Autodesk Inventor part; units mm, degrees
ref_plane "YZ Plane" through (0, 0, 0) normal (1, 0, 0) x (0, 1, 0)
ref_plane "XZ Plane" through (0, 0, 0) normal (0, 1, 0) x (-1, 0, 0)
ref_plane "XY Plane" through (0, 0, 0) normal (0, 0, 1) x (1, 0, 0)
sketch "Sketch1" plane through (0, 0, 0) normal (0, 1, 0) x (-1, 0, 0)
  arc A0 (176.3419, -210.5927) -> (175.3044, -30.5987) centre (175.3044, -120.5987) ccw
  line L0 (175.3044, -30.5987) -> (91.4725, -30.5987)
  line L1 (-2.1956, -66.2894) -> (-2.1956, -174.8751)
  line L2 (91.4505, -210.5927) -> (176.3419, -210.5927)
  arc A1 (44.9453, -8.483) -> (-6.6956, -55.5772) centre (17.8044, -30.5822) ccw
  arc A2 (-6.6956, -185.5872) -> (44.9372, -232.6914) centre (17.8044, -210.5822) ccw
  line L3 (265.3044, -138.5987) -> (263.4861, -138.5987)
  line L4 (263.4861, -102.5987) -> (265.3044, -102.5987)
  circle A3 centre (175.3044, -120.5987) radius 14.5
  line L5 (175.3044, -52.5987) -> (77.8044, -52.5987)
  line L6 (77.8044, -188.5987) -> (175.3044, -188.5987)
  arc A4 (237.9792, -94.2194) -> (175.3044, -52.5987) centre (175.3044, -120.5987) ccw
  arc A5 (175.3044, -188.5987) -> (237.9792, -146.978) centre (175.3044, -120.5987) ccw
  line L7 (228.7624, -133.0987) -> (217.1374, -133.0987)
  line L8 (217.1374, -108.0987) -> (228.7624, -108.0987)
  line L9 (139.9491, -108.0987) -> (106.0335, -108.0987)
  line L10 (106.0335, -133.0987) -> (139.9491, -133.0987)
  arc A6 (208.3305, -102.8356) -> (139.9491, -108.0987) centre (175.3044, -120.5987) ccw
  arc A7 (139.9491, -133.0987) -> (208.3305, -138.3619) centre (175.3044, -120.5987) ccw
  line L11 (62.8044, -67.5987) -> (62.8044, -62.504)
  line L12 (62.8044, -178.6935) -> (62.8044, -173.5987)
  arc A8 (106.0335, -108.0987) -> (74.0544, -77.0277) centre (62.8044, -120.5987) ccw
  arc A9 (74.0544, -164.1698) -> (106.0335, -133.0987) centre (62.8044, -120.5987) ccw
  circle A10 centre (62.8044, -120.5987) radius 21
  circle A11 centre (17.8044, -30.5822) radius 21
  circle A12 centre (17.8044, -210.5822) radius 21
  arc A13 (239.6919, -108.0987) -> (241.6431, -105.6593) centre (239.6919, -106.0987) ccw
  arc A14 (228.7624, -108.0987) -> (237.9792, -94.2194) centre (228.7624, -98.0987) ccw
  arc A15 (208.3305, -102.8356) -> (217.1374, -108.0987) centre (217.1374, -98.0987) ccw
  arc A16 (217.1374, -133.0987) -> (208.3305, -138.3619) centre (217.1374, -143.0987) ccw
  arc A17 (237.9792, -146.978) -> (228.7624, -133.0987) centre (228.7624, -143.0987) ccw
  arc A18 (77.8044, -52.5987) -> (62.8044, -67.5987) centre (77.8044, -67.5987) ccw
  arc A19 (62.8044, -173.5987) -> (77.8044, -188.5987) centre (77.8044, -173.5987) ccw
  arc A20 (62.8044, -62.504) -> (74.0544, -77.0277) centre (77.8044, -62.504) ccw
  arc A21 (74.0544, -164.1698) -> (62.8044, -178.6935) centre (77.8044, -178.6935) ccw
  arc A22 (44.9453, -8.483) -> (91.4725, -30.5987) centre (91.4725, 29.4013) ccw
  arc A23 (91.4505, -210.5927) -> (44.9372, -232.6914) centre (91.4505, -270.5927) ccw
  arc A24 (-2.1956, -66.2894) -> (-6.6956, -55.5772) centre (-17.1956, -66.2894) ccw
  arc A25 (-6.6956, -185.5872) -> (-2.1956, -174.8751) centre (-17.1956, -174.8751) ccw
  point P0 (0, 0)
  point P1 (-2.1956, -181.8594)
  point P2 (242.1457, -108.0987)
  point P3 (242.1457, -133.0987)
  point P4 (62.8044, -188.5987)
  point P5 (210.6598, -108.0987)
  point P6 (210.6598, -133.0987)
  point P7 (62.8044, -52.5987)
  point P8 (62.8044, -75.5987)
  point P9 (62.8044, -165.5987)
  point P10 (-2.1956, -59.3051)
  point P11 (52.8044, -30.5987)
  point P12 (52.8044, -210.5927)
  point P13 (63.0223, -65.0513)
  point P14 (63.0223, -176.1461)
  dimension "d0" = 180
  dimension "d1" = 20
  dimension "d2" = 20
  dimension "d3" = 42
  dimension "d4" = 70
  dimension "d5" = 42
  dimension "d6" = 70
  dimension "d7" = 112.5
  dimension "d8" = 90
  dimension "d9" = 90
  dimension "d10" = 25
  dimension "d11" = 90
  dimension "d12" = 68
  dimension "d13" = 77.5
  dimension "d14" = 37.5
  dimension "d15" = 37.5
  dimension "d16" = 29
  dimension "d17" = 45
  dimension "d18" = 45
  dimension "d19" = 42
  dimension "d20" = 25
  dimension "d21" = 77.5
  dimension "d22" = 112.5
  dimension "d23" = 112.5
  dimension "d24" = 45
  dimension "d25" = 68
  dimension "d26" = 2
  dimension "d27" = 10
  dimension "d28" = 15
  dimension "d29" = 60
extrude "Extrusion1" add sketch "Sketch1" along normal blind 10
equation "\"d2\" = d1"
equation "\"d5\" = d3"
equation "\"d6\" = d4"
equation "\"d15\" = d14"
equation "\"d18\" = d17"
equation "\"d20\" = d10"
equation "\"d21\" = d13"
equation "\"d25\" = d12"
For this review, take the finished solid that the model builds, in its own axes (mm). A direction names the side the tool comes from. Give positions to 0.01 mm unless a question says otherwise; leave off trailing zeros. Order: outer loops, then holes, each group sorted by start corner. A loop starts at its lowest first (then second) coordinate and runs counter-clockwise, first axis right, second up. Notation, with made-up numbers: (-13.75, 64.25) - (24.25, 64.25) arc R22 ccw to (24.25, 70.25) - close; hole circle Ø7 at (-19.5, 62). An arc over 180 degrees is marked (long way). Answer as a JSON object with one key per item and string values. Group by question number.
Item 1: Clearance check with flat-ended pins moving along their axes: pin 1 Ø5 at (x, y) = (-122, 7) entering from -Z; pin 2 Ø6 at (y, z) = (4, -91.5) entering from +X; pin 3 Ø1 at (x, y) = (-59.5, 3) entering from -Z. State where each tip first meets the part, or that it passes through.
Item 2: Machinability: for faces 1 (the flat face through (-223, 5, -133.099)), 2 (the cylindrical face through (-65.366, 4.93, -216.559)), 3 (the cylindrical face through (3.334, 4.93, -180.607)), 4 (the flat face through (-134, 5, -30.599)), which of the approach directions +Z, -Z, +X, -X, +Y, -Y give a long, thin tool a straight path to every point of the face, cutting with its end or side? Answer none if there is none.
Item 3: Wall thickness on line 1 along Z through (x, y) = (-112, 8.75); line 2 along X through (y, z) = (6, -106); line 3 along Z through (x, y) = (-232.5, 1.75): over which ranges is each line inside the solid? List them lowest first.
Item 4: Take a section at A-A on x = -150. Give the boundary of the cut face in (y, z), and give its area (3 significant figures).
Item 5: Draft analysis for pull direction Z (two halves, no side actions). For faces 5 (the flat face through (-91, 10, -119)), 6 (the cylindrical face through (3.4, 4.9, -60.4)), 7 (the cylindrical face through (-265.27, 4.93, -118.11)), state which applies: pulls with the +Z half, pulls with the -Z half, needs draft (parallel to the pull), parting line crosses it, or undercut.
Item 6: Take a section at B-B on z = -151. Give the boundary of the cut face in (x, y).
Item 7: Take a section at C-C on z = -25. Give the boundary of the cut face in (x, y), and give its area (3 significant figures).
Reported:
{
 "1": {"pin 1": "z = -210.59", "pin 2": "x = 2.2", "pin 3": "z = -220.13"},
 "2": {"face 1": "+Y, -Y", "face 2": "-Z, -X, +Y, -Y", "face 3": "+X, +Y, -Y", "face 4": "+Z, -X, +Y, -Y"},
 "3": {"line 1": "-210.59 to -188.6, -133.1 to -108.1, -52.6 to -30.6", "line 2": "-264.11 to -234.89, -211.01 to -140.76, -105.37 to -77.9, -47.71 to 2.2", "line 3": "-190.09 to -157.38, -133.82 to -107.37, -83.82 to -51.11"},
 "4": {"outline": "(0, -210.59) - (10, -210.59) - (10, -188.6) - (0, -188.6) - close; (0, -148.27) - (10, -148.27) - (10, -92.92) - (0, -92.92) - close; (0, -52.6) - (10, -52.6) - (10, -30.6) - (0, -30.6) - close", "area": "993 mm^2"},
 "5": {"face 5": "needs draft", "face 6": "undercut", "face 7": "parting line crosses it"},
 "6": {"outline": "(-260.01, 0) - (-236.13, 0) - (-236.13, 10) - (-260.01, 10) - close; (-197.26, 0) - (-153.35, 0) - (-153.35, 10) - (-197.26, 10) - close; (-95.98, 0) - (2.2, 0) - (2.2, 10) - (-95.98, 10) - close"},
 "7": {"outline": "(-66.16, 0) - (-38.05, 0) - (-38.05, 10) - (-66.16, 10) - close; (2.44, 0) - (16.75, 0) - (16.75, 10) - (2.44, 10) - close", "area": "424 mm^2"}
}
